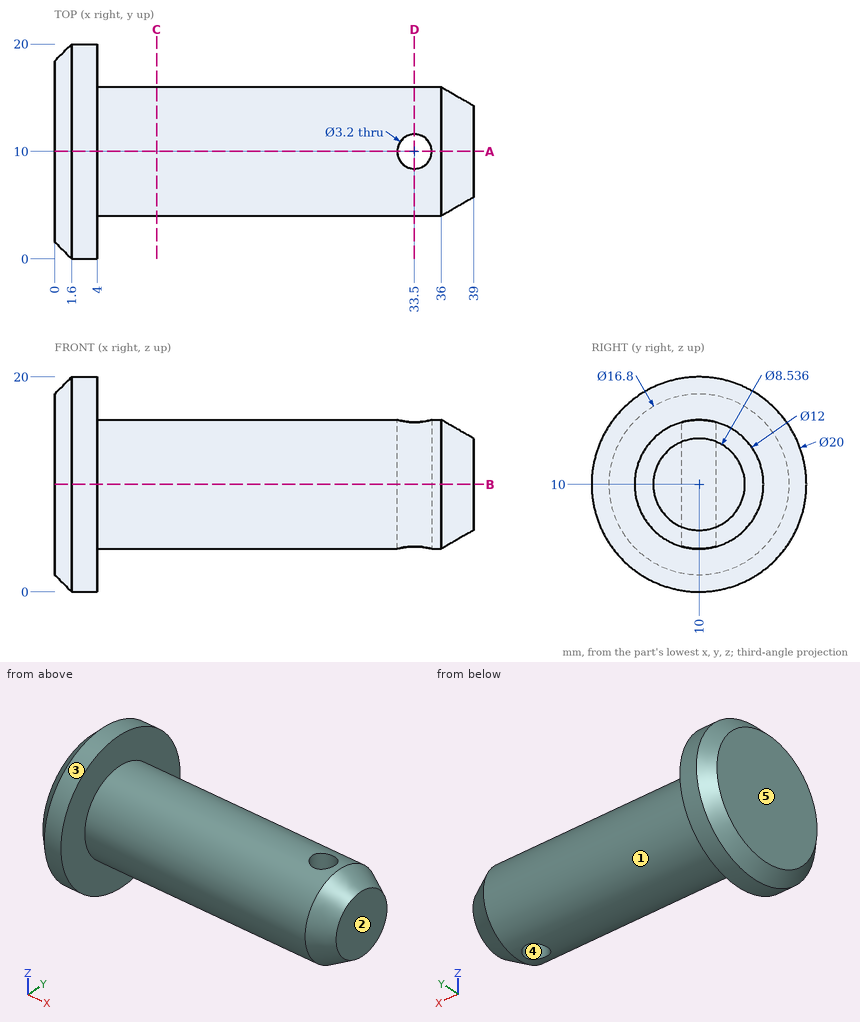
Job drawing, mm, ordinate dimensions from the low corner. One solid piece. A direction names the side the tool comes from. Give positions to 0.01 mm unless a question says otherwise; leave off trailing zeros. Write each loop counter-clockwise with the first axis right and the second up, starting at its lowest first coordinate (ties: lowest second). Pieces come first, ordered by that corner, then holes. Notation, with made-up numbers: (51.25, 87) - (69.25, 87) arc R21 cw to (69.25, 119) - close; hole circle Ø1 at (83, -19). An arc over 180 degrees is marked (long way). Answer as CSV lines item,"result".
1. Two-plate mould, pull along Y, no slides. Class the marked faces 3, 4 and 5: +Y half, -Y half, draft (parallel to the pull), parting line (faces both ways), or undercut.
Responses:
face 3,"parting line"
face 4,"undercut"
face 5,"draft"
2. Drill centre lines: L1, parallel to X at y = 10, z = 9; L2, parallel to X at y = 11.5, z = 1.75; L3, parallel to X at y = 11.25, z = 7.75. Where is each one in solid material? Low to high. Write a range as [from, to].
Responses:
L1,"x = [0, 31.9], [35.1, 39]"
L2,"x = [0, 4]"
L3,"x = [0, 32.5], [34.5, 39]"
3. Band-saw the part on C-C (x = 9.5). Write the cut outline in (y, z).
Responses:
outline,"circle Ø12 at (10, 10)"
4. 3-axis set-ups, long thin cutter, end or side, ignore diameter. For the marked faces 1 and 2: which of +Z, -Z, +X, -X, +Y, -Y reach the whole face in a straight line?
Responses:
face 1,"+X"
face 2,"+Z, -Z, +X, +Y, -Y"
5. Band-saw the part on B-B (z = 10). Write the cut outline in (x, y).
Responses:
outline,"(0, 1.6) - (1.6, 0) - (4, 0) - (4, 4) - (36, 4) - (39, 5.73) - (39, 14.27) - (36, 16) - (4, 16) - (4, 20) - (1.6, 20) - (0, 18.4) - close; hole circle Ø3.2 at (33.5, 10)"
6. Band-saw the part on A-A (y = 10). Write the cut outline in (x, z).
Responses:
outline,"(0, 1.6) - (1.6, 0) - (4, 0) - (4, 4) - (31.9, 4) - (31.9, 16) - (4, 16) - (4, 20) - (1.6, 20) - (0, 18.4) - close; (35.1, 4) - (36, 4) - (39, 5.73) - (39, 14.27) - (36, 16) - (35.1, 16) - close"
7. Band-saw the part on D-D (x = 33.5). Write the cut outline in (y, z).
Responses:
outline,"(8.4, 4.22) - (8.4, 15.78) arc R6 ccw to start; (11.6, 4.22) arc R6 ccw to (11.6, 15.78) - close"
8. Pin check, flat tips, straight feed: pin 1 (3 mm diameter, centred on x = 33.5, y = 10, fed in from -Z); pin 2 (6 mm diameter, centred on y = 4.5, z = 3, fed in from +X); pin 3 (6 mm diameter, centred on x = 34.5, z = 16, fed in from -Y); pin 4 (1 mm diameter, centred on x = 31, z = 4.5, fed in from -Y). Stop position of each tip, or through.
Responses:
pin 1,"passes through"
pin 2,"stops at x = 36.17"
pin 3,"stops at y = 4.8"
pin 4,"stops at y = 6.68"
